```python
from build123d import *

# Parameters (mm, degrees)
ESBO_O1_W                = 8
ESBO_O1_H                = 2
RESSALTO_EXTRUS_O1_DEPTH = 10
CORTE_EXTRUS_O1_REACH    = 74.966
ESBO_O4_W                = 20
ESBO_O4_H                = 15
ESBO_O4_R                = 2
RESSALTO_EXTRUS_O2_DEPTH = 5


with BuildPart() as part:
    # Esboço1 → Ressalto-extrusão1 (new, symmetric)
    with BuildSketch(Plane(origin=(0, 0, 0), x_dir=(0, 0, -1), z_dir=(1, 0, 0))):
        Polygon((-35, 18), (-10, 18), (-10, 5), (10, 5), (10, 18), (35, 18), (35, 0), (-35, 0), align=None)
        with Locations((-22.5, 4)):
            Rectangle(ESBO_O1_W, ESBO_O1_H, mode=Mode.SUBTRACT)
        with Locations((22.5, 4)):
            Rectangle(ESBO_O1_W, ESBO_O1_H, mode=Mode.SUBTRACT)
    extrude(amount=RESSALTO_EXTRUS_O1_DEPTH, both=True)

    # Corte-extrusão1: up to this face of the body (flat: up to its plane)
    corte_extrus_o1_end = Plane(part.part.faces().sort_by_distance((0, 9, -35))[0])
    # Esboço2 → Corte-extrusão1 (cut, up to the picked face)
    with BuildSketch(Plane.XY.offset(35), mode=Mode.PRIVATE) as corte_extrus_o1_sk1:
        with BuildLine():
            Line((-10, 15), (-6.873863542, 15))
            ThreePointArc((-6.873863542, 15), (0, 10.5), (6.873863542, 15))
            Line((6.873863542, 15), (10, 15))
            Line((10, 15), (10, 18))
            Line((10, 18), (7.5, 18))
            Line((7.5, 18), (-7.5, 18))
            Line((-7.5, 18), (-10, 18))
            Line((-10, 18), (-10, 15))
        make_face()
    corte_extrus_o1_tool1 = split(extrude(corte_extrus_o1_sk1.sketch, amount=-CORTE_EXTRUS_O1_REACH, mode=Mode.PRIVATE), bisect_by=corte_extrus_o1_end, keep=Keep.BOTH, mode=Mode.PRIVATE)
    add(corte_extrus_o1_tool1.solids().sort_by(Axis((0, 15.069195, 35), (0, 0, -1)))[0], mode=Mode.SUBTRACT)

    # Esboço4 → Ressalto-extrusão2 (add)
    # profile 1 of 2: a face of its own
    with BuildSketch(Plane(origin=(0, 5, 0), x_dir=(1, 0, 0), z_dir=(0, 1, 0))):
        with Locations((0, 42.5)):
            Rectangle(ESBO_O4_W, ESBO_O4_H)
        with Locations(Location((0, 42.5, 0), (0, 0, 270))):
            Circle(ESBO_O4_R, mode=Mode.SUBTRACT)
    # profile 2 of 2: a face of its own
    with BuildSketch(Plane(origin=(0, 5, 0), x_dir=(1, 0, 0), z_dir=(0, 1, 0))):
        with Locations((0, -42.5)):
            Rectangle(ESBO_O4_W, ESBO_O4_H)
        with Locations(Location((0, -42.5, 0), (0, 0, 270))):
            Circle(ESBO_O4_R, mode=Mode.SUBTRACT)
    extrude(amount=-RESSALTO_EXTRUS_O2_DEPTH)


solid = part.part
```
Here's how the part is built. I have some questions about the finished solid (model axes, mm). A direction names the side the tool comes from. Coordinates: 2 decimals unless noted, no trailing zeros. Order: outer loops, then holes, each group sorted by start corner. A loop starts at its lowest first (then second) coordinate and runs counter-clockwise, first axis right, second up. Notation, with made-up numbers: M 71.5,-26 L 109.5,-26 A4 ccw 109.5,-21 Z; hole C -25,23.25 d6. An arc over 180 degrees is marked long. Answer as a JSON object with one key per item and string values. Group by question number.
(1) Suppose I cut it at D-D, the plane z = -9. Please give me the cut outline in (x, y), then the cut area to 3 significant figures.
(2) For pin 1 (8 mm diameter, centred on x = -4, y = 11.5, fed in from -Z); pin 2 (7.5 mm diameter, centred on x = -3.5, z = 46, fed in from +Y); pin 3 (5 mm diameter, centred on x = 4, y = 8.5, fed in from +Z), each with a flat end and sliding along its axis, tell me the tip position at first contact or that it passes through.
(3) I need wall thicknesses on probe 1 along Z at (x, y) = (3.5, 4.5); probe 2 along Z at (x, y) = (-3, 7.25); probe 3 along X at (y, z) = (3.6, -42.5). Which ranges of each line are inside material? Lowest first, please.
(4) If we mould it in two halves opening along Z, with no side actions, what happens to faces 1 (the face through (-10, 4, 1)), 2 (the face through (0, 9, 10)), 3 (the face through (0, 3, 50))? For each: released by +Z, released by -Z, zero draft, split by the parting line, or undercut.
(5) Suppose I cut it at A-A, the plane z = -42.5. Please give me the cut outline in (x, y), then the cut area to 3 significant figures.
(6) Which directions (+Z, -Z, +X, -X, +Y, -Y) give clear straight access to the entire face, cutting with the end or side of a thin tool? Please do faces 4 (the face through (0, 3, 23)), 5 (the face through (-0.1, 10.5, 22.7)), 6 (the face through (0, 9, -35)).
(7) Suppose I cut it at B-B, the plane x = 0. Please give me the cut outline in (y, z).
(8) Suppose I cut it at C-C, the plane x = 5.5. Please give me the cut outline in (y, z), then the cut area to 3 significant figures.
Values found:
{
 "1": {"outline": "M -10,0 L 10,0 L 10,5 L -10,5 Z", "area": "100 mm^2"},
 "2": {"pin 1": "stops at z = -35", "pin 2": "stops at y = 5", "pin 3": "stops at z = 35"},
 "3": {"probe 1": "z = -50 to -26.5, -18.5 to 18.5, 26.5 to 50", "probe 2": "z = -35 to -10, 10 to 35", "probe 3": "x = -10 to -2, 2 to 10"},
 "4": {"face 1": "zero draft", "face 2": "undercut", "face 3": "released by +Z"},
 "5": {"outline": "M -10,0 L -2,0 L -2,5 L -10,5 Z; M 2,0 L 10,0 L 10,5 L 2,5 Z", "area": "80.0 mm^2"},
 "6": {"face 4": "+X, -X", "face 5": "+Z, -Z, +Y", "face 6": "-Z, +X, -X, +Y"},
 "7": {"outline": "M 0,-50 L 5,-50 L 5,-44.5 L 0,-44.5 Z; M 0,-40.5 L 5,-40.5 L 5,-35 L 10.5,-35 L 10.5,-10 L 5,-10 L 5,10 L 10.5,10 L 10.5,35 L 5,35 L 5,40.5 L 0,40.5 Z; M 0,44.5 L 5,44.5 L 5,50 L 0,50 Z; hole M 3,-26.5 L 5,-26.5 L 5,-18.5 L 3,-18.5 Z; hole M 3,18.5 L 5,18.5 L 5,26.5 L 3,26.5 Z"},
 "8": {"outline": "M 0,-50 L 5,-50 L 5,-35 L 12.9,-35 L 12.9,-10 L 5,-10 L 5,10 L 12.9,10 L 12.9,35 L 5,35 L 5,50 L 0,50 Z; hole M 3,-26.5 L 5,-26.5 L 5,-18.5 L 3,-18.5 Z; hole M 3,18.5 L 5,18.5 L 5,26.5 L 3,26.5 Z", "area": "863 mm^2"}
}
